Here's how the part is built. I have some questions about the finished solid (model axes, mm). A direction names the side the tool comes from. Round coordinates to 2 decimals unless told otherwise and drop trailing zeros. Order: outer loops, then holes, each group sorted by start corner. A loop starts at its lowest first (then second) coordinate and runs counter-clockwise, first axis right, second up. Notation, with made-up numbers: M 86.25,52 L 128.25,52 A29 cw 128.25,89 Z; hole C -13.75,82.5 d1. An arc over 180 degrees is marked long. Write each question's results on one line, items separated by ' | '. Start each with the question number.
```python
from build123d import *

# Parameters (mm, degrees)
CROQUIS2_R              = 1.5
SALIENTE_EXTRUIR1_DEPTH = 2.5
CORTAR_EXTRUIR1_DEPTH   = 2.5
REDONDEO1_R             = 2
SALIENTE_EXTRUIR2_DEPTH = 2.5


with BuildPart() as part:
    # Croquis2 → Saliente-Extruir1 (new body)
    with BuildSketch(Plane.XY):
        with BuildLine():
            Line((-97.318076, 19.5), (-30.318076, 19.5))
            ThreePointArc((-30.318076, 19.5), (-26.318076, 15.5), (-30.318076, 11.5))
            ThreePointArc((-30.318076, 11.5), (-41.818076, 0), (-30.318076, -11.5))
            ThreePointArc((-30.318076, -11.5), (-26.318076, -15.5), (-30.318076, -19.5))
            Line((-30.318076, -19.5), (-97.318076, -19.5))
            ThreePointArc((-97.318076, -19.5), (-100.146503125, -18.328427125), (-101.318076, -15.5))
            Line((-101.318076, -15.5), (-101.318076, 15.5))
            ThreePointArc((-101.318076, 15.5), (-100.146503125, 18.328427125), (-97.318076, 19.5))
        make_face()
        with Locations((-97.318076, 15.5)):
            Circle(CROQUIS2_R, mode=Mode.SUBTRACT)
        with Locations((-30.318076, 15.5)):
            Circle(CROQUIS2_R, mode=Mode.SUBTRACT)
        with Locations((-30.318076, -15.5)):
            Circle(CROQUIS2_R, mode=Mode.SUBTRACT)
        with Locations((-97.318076, -15.5)):
            Circle(CROQUIS2_R, mode=Mode.SUBTRACT)
    extrude(amount=SALIENTE_EXTRUIR1_DEPTH)

    # Croquis3 → Cortar-Extruir1 (cut)
    with BuildSketch(Plane.XY.offset(2.5)):
        Polygon((-67.818076, 3), (-41.818076, 15.5), (-93.818076, 15.5), align=None)
        Polygon((-67.818076, -3), (-93.818076, -15.5), (-41.818076, -15.5), align=None)
        Polygon((-70.818076, 0), (-95.228698469, 11.735876187), (-95.228698469, -11.735876187), align=None)
    extrude(amount=-CORTAR_EXTRUIR1_DEPTH, mode=Mode.SUBTRACT)

    # Redondeo1
    redondeo1_edges = [part.edges().sort_by_distance(p)[0] for p in [
        (-67.818076, -3, 1.25),
        (-41.818076, -15.5, 1.25),
        (-93.818076, -15.5, 1.25),
        (-70.818076, 0, 1.25),
        (-95.228698469, -11.735876187, 1.25),
        (-95.228698469, 11.735876187, 1.25),
        (-67.818076, 3, 1.25),
        (-93.818076, 15.5, 1.25),
        (-41.818076, 15.5, 1.25),
    ]]
    fillet(redondeo1_edges, radius=REDONDEO1_R)

    # Croquis5 → Saliente-Extruir2 (add)
    with BuildSketch(Plane.XY.offset(2.5)):
        with BuildLine():
            Line((-97.318076, 19.5), (-30.318076, 19.5))
            ThreePointArc((-30.318076, 19.5), (-63.818076, 27.5), (-97.318076, 19.5))
        make_face()
        with BuildLine():
            Line((-97.318076, -19.5), (-30.318076, -19.5))
            ThreePointArc((-30.318076, -19.5), (-63.818076, -27.5), (-97.318076, -19.5))
        make_face()
    extrude(amount=-SALIENTE_EXTRUIR2_DEPTH)


solid = part.part
```
(1) I'm going to push flat-ended pins straight in: pin 1 Ø1.8 at (x, y) = (-97.32, 15.5) entering from -Z; pin 2 Ø1 at (x, z) = (-60.5, 2) entering from -Y; pin 3 Ø1.5 at (x, z) = (-36.5, 2) entering from +Y. Where does each tip first touch, or does it pass through?
(2) Please list where these lines run through material, in increasing order: line 1 (Y direction, x = -80.5, z = 2.45); line 2 (Y direction, x = -52.5, z = 2.35); line 3 (Y direction, x = -55.5, z = 1.3).
(3) I want a section at B-B on x = -75.5. Write out the boundary of the cut face in (y, z), and give its area (3 significant figures).
(4) On a 3-axis mill with a long thin cutter (end or side, diameter ignored), from which of +Z, -Z, +X, -X, +Y, -Y can I reach the whole of each face in a straight line? I mean faces 1 (the flat face through (-77.18, -7.5, 1.27)), 2 (the cylindrical face through (-63.3, 27.5, 1.3)). Say none if no direction works.
(5) I want a section at D-D on x = -66. Write out the boundary of the cut face in (y, z).
(6) I want a section at C-C on z = 1.15. Give the number of separate pieces and of enclosed holes in the cut face, and give its area (3 significant figures).
(7) If we mould it in two halves opening along Y, with no side actions, what happens to faces 3 (the cylindrical face through (-100.115, -18.359, 1.232)), 4 (the cylindrical face through (-73.434, -0.031, 1.232)), 5 (the flat face through (-64, 0, 0))? For each: pulls with the +Y half, pulls with the -Y half, needs draft (parallel to the pull), parting line crosses it, or undercut.
(8) I want a section at A-A on y = 0. Write out the boundary of the cut face in (x, z).
Solutions:
1) pin 1: through | pin 2: y = -27.45 | pin 3: y = 22.58
2) line 1: -25.6 to -15.5, -9.1 to -4.65, 4.65 to 9.1, 15.5 to 25.6 | line 2: -26.63 to -15.5, -10.36 to 10.36, 15.5 to 26.63 | line 3: -27.03 to -15.5, -8.92 to 8.92, 15.5 to 27.03
3) outline: M -26.57,0 L -15.5,0 L -15.5,2.5 L -26.57,2.5 Z; M -6.69,0 L -2.25,0 L -2.25,2.5 L -6.69,2.5 Z; M 2.25,0 L 6.69,0 L 6.69,2.5 L 2.25,2.5 Z; M 15.5,0 L 26.57,0 L 26.57,2.5 L 15.5,2.5 Z | area: 77.6 mm^2
4) face 1: +Z, -Z | face 2: +Z, -Z, +Y
5) outline: M -27.47,0 L -15.5,0 L -15.5,2.5 L -27.47,2.5 Z; M -3.87,0 L 3.87,0 L 3.87,2.5 L -3.87,2.5 Z; M 15.5,0 L 27.47,0 L 27.47,2.5 L 15.5,2.5 Z
6) separate pieces: 1 | enclosed holes: 7 | area: 2,420 mm^2
7) face 3: pulls with the -Y half | face 4: undercut | face 5: needs draft
8) outline: M -101.32,0 L -95.23,0 L -95.23,2.5 L -101.32,2.5 Z; M -73.43,0 L -41.82,0 L -41.82,2.5 L -73.43,2.5 Z
